from build123d import *

# Parameters (mm, degrees)
F0_W     = 25.4
F0_H     = 12.7
F1_DEPTH = 1
F3_D     = 2.032
F4_W     = 4
F4_H     = 12.7
F5_DEPTH = 0.25
F6_W     = 1.55
F6_H     = 12.7
F7_DEPTH = 0.5
F8_W     = 1.55
F8_H     = 10
F9_DEPTH = 0.25


with BuildPart() as f1:
    # F0 (on Front) → F1 (new body)
    with BuildSketch(Plane.XZ):
        Rectangle(F0_W, F0_H)
    extrude(amount=F1_DEPTH)

    # F3 (through all)
    with Locations(Plane(origin=(0, 0, 0), x_dir=(1, 0, 0), z_dir=(0, 1, 0))):
        with Locations((-7.239, 3.2512), (7.239, 3.2512), (7.239, -3.2512), (-7.239, -3.2512)):
            Hole(F3_D / 2)

    # F4 (on Front) → F5 (cut)
    with BuildSketch(Plane.XZ):
        Rectangle(F4_W, F4_H)
    extrude(amount=F5_DEPTH, mode=Mode.SUBTRACT)

    # F6 (on face) → F7 (cut)
    with BuildSketch(Plane.XZ.offset(1)):
        Rectangle(F6_W, F6_H)
    extrude(amount=-F7_DEPTH, mode=Mode.SUBTRACT)

    # F8 (on face) → F9 (cut)
    with BuildSketch(Plane.XZ.offset(0.5)):
        Rectangle(F8_W, F8_H)
    extrude(amount=-F9_DEPTH, mode=Mode.SUBTRACT)


solid = f1.part
Build history of the part. All positions in model axes, mm. A direction names the side the tool comes from. Give positions to 0.01 mm unless a question says otherwise; leave off trailing zeros. Write each loop counter-clockwise with the first axis right and the second up, starting at its lowest first coordinate (ties: lowest second). Pieces come first, ordered by that corner, then holes. Notation, with made-up numbers: (48.5, 31) - (105.5, 31) arc R22 ccw to (105.5, 54) - close; hole circle Ø3 at (-16, 55). An arc over 180 degrees is marked (long way). Use one line per item in the form item = value. Start each with the question number.
1. Band-saw the part on A-A on y = -0.7. Write the cut outline in (x, z) (3 decimals).
2. Band-saw the part on C-C on z = 3.75. Write the cut outline in (x, y) (3 decimals), plus the area to 3 significant figures.
3. Two-plate mould, pull along Z, no slides. Class faces 1 (the face through (8.254, -0.507, 3.207)), 2 (the face through (-1, -0.25, 0)), 3 (the face through (2.6, -0.5, 6.35)): released by +Z, released by -Z, zero draft, split by the parting line, or undercut.
4. Band-saw the part on D-D on x = 7.75. Write the cut outline in (y, z), plus the area to 3 significant figures.
5. 3-axis set-ups, long thin cutter, end or side, ignore diameter. For faces 4 (the face through (7, -1, 0)), 5 (the face through (0, -0.5, -6)): which of +Z, -Z, +X, -X, +Y, -Y reach the whole face in a straight line?
6. Probe line 1 (X direction, y = -0.85, z = -3.25) (3 decimals); line 2 (Z direction, x = 7, y = -0.7); line 3 (X direction, y = -0.6, z = 6.25) (3 decimals). List the from-to ranges inside material, lowest first. Write a range as [from, to].
7. Band-saw the part on B-B on z = -4.75. Write the cut outline in (x, y) (3 decimals), plus the area to 3 significant figures.
Conclusion:
q1.outline = (-12.7, -6.35) - (-0.775, -6.35) - (-0.775, 6.35) - (-12.7, 6.35) - close; (0.775, -6.35) - (12.7, -6.35) - (12.7, 6.35) - (0.775, 6.35) - close; hole circle Ø2.032 at (-7.239, -3.251); hole circle Ø2.032 at (-7.239, 3.251); hole circle Ø2.032 at (7.239, -3.251); hole circle Ø2.032 at (7.239, 3.251)
q2.outline = (-12.7, -1) - (-8.124, -1) - (-8.124, 0) - (-12.7, 0) - close; (-6.354, -1) - (-0.775, -1) - (-0.775, -0.25) - (-2, -0.25) - (-2, 0) - (-6.354, 0) - close; (0.775, -1) - (6.354, -1) - (6.354, 0) - (2, 0) - (2, -0.25) - (0.775, -0.25) - close; (8.124, -1) - (12.7, -1) - (12.7, 0) - (8.124, 0) - close
q2.area = 19.7 mm²
q3.face_1 = undercut
q3.face_2 = zero draft
q3.face_3 = released by +Z
q4.outline = (-1, -6.35) - (0, -6.35) - (0, -4.13) - (-1, -4.13) - close; (-1, -2.37) - (0, -2.37) - (0, 2.37) - (-1, 2.37) - close; (-1, 4.13) - (0, 4.13) - (0, 6.35) - (-1, 6.35) - close
q4.area = 9.19 mm²
q5.face_4 = +Z, -Z, +X, -X, -Y
q5.face_5 = +Z, -Z, -Y
q6.line_1 = [-12.7, -8.255], [-6.223, -0.775], [0.775, 6.223], [8.255, 12.7]
q6.line_2 = [-6.35, -4.24], [-2.26, 2.26], [4.24, 6.35]
q6.line_3 = [-12.7, -0.775], [0.775, 12.7]
q7.outline = (-12.7, -1) - (-0.775, -1) - (-0.775, -0.25) - (-2, -0.25) - (-2, 0) - (-12.7, 0) - close; (0.775, -1) - (12.7, -1) - (12.7, 0) - (2, 0) - (2, -0.25) - (0.775, -0.25) - close
q7.area = 23.2 mm²
